Geometry check sheet. Reference: the model listing, model coordinates, mm. A direction names the side the tool comes from. Coordinates: 2 decimals unless noted, no trailing zeros. Loops run counter-clockwise (first coordinate to the right, second up) from the corner with the lowest first, then second, coordinate; pieces in that order, holes last.
from build123d import *

# Parameters (mm, degrees)
SM_BASE_FLANGE_1_DEPTH   = 41
SKETCH_9_R               = 2.5
CUT_EXTRUDE_4_DEPTH      = 61.6465168
CUT_EXTRUDE_5_DEPTH      = 78.103826105
CUT_EXTRUDE_5_DEPTH_BACK = 78.103826105
SKETCH_10_R              = 2.5


# Sheet-metal steps are written as plain solids
with BuildPart() as part:
    # Sketch 1 → Базовая кромка1 (new body)
    with BuildSketch(Plane.XY):
        with BuildLine():
            Line((-25, 30), (-25, 1))
            ThreePointArc((-25, 1), (-24.707106781, 0.292893219), (-24, 0))
            Line((-24, 0), (24, 0))
            ThreePointArc((24, 0), (24.707106781, 0.292893219), (25, 1))
            Line((25, 1), (25, 30))
            Line((25, 30), (29, 30))
            Line((29, 30), (29, 1))
            ThreePointArc((29, 1), (27.535533906, -2.535533906), (24, -4))
            Line((24, -4), (-24, -4))
            ThreePointArc((-24, -4), (-27.535533906, -2.535533906), (-29, 1))
            Line((-29, 1), (-29, 30))
            Line((-29, 30), (-25, 30))
        make_face()
    extrude(amount=SM_BASE_FLANGE_1_DEPTH)

    # Эскиз9 → Вырез-Вытянуть4 (cut, through all)
    with BuildSketch(Plane.XZ.offset(4)):
        with Locations((-18, 20.5)):
            Circle(SKETCH_9_R)
        with Locations((-9, 36.088457268)):
            Circle(SKETCH_9_R)
        with Locations((9, 36.088457268)):
            Circle(SKETCH_9_R)
        with Locations((18, 20.5)):
            Circle(SKETCH_9_R)
        with Locations((9, 4.911542732)):
            Circle(SKETCH_9_R)
        with Locations((-9, 4.911542732)):
            Circle(SKETCH_9_R)
    extrude(amount=-CUT_EXTRUDE_4_DEPTH, mode=Mode.SUBTRACT)

    # Эскиз10 → Вырез-Вытянуть5 (cut, two sides: drawn at the far end of the back side and taken through both)
    with BuildSketch(Plane(origin=(29, 0, 0), x_dir=(0, 0, -1), z_dir=(1, 0, 0)).offset(-CUT_EXTRUDE_5_DEPTH_BACK)):
        with Locations((-33, 25)):
            Circle(SKETCH_10_R)
        with Locations((-20.5, 25)):
            Circle(SKETCH_10_R)
        with Locations((-8, 25)):
            Circle(SKETCH_10_R)
        with Locations((-20.5, 12.5)):
            Circle(SKETCH_10_R)
    extrude(amount=CUT_EXTRUDE_5_DEPTH + CUT_EXTRUDE_5_DEPTH_BACK, mode=Mode.SUBTRACT)


solid = part.part
1) Mould release check, pull along X, two halves, no side actions. Record for faces 3 (the cylindrical face through (16, -2, 22)), 4 (the cylindrical face through (-27, -3, 20)), 5 (the flat face through (0, -1, 0)): +X half, -X half, draft (parallel to the pull), parting line (faces both ways), or undercut.
Data:
face 3: undercut
face 4: -X half
face 5: draft
2) Access from +Z, -Z, +X, -X, +Y, -Y to the whole of each face (thin tool, end or side, straight path). Record for faces 1 (the cylindrical face through (27, 11, 22.5)), 2 (the flat face through (25, 15.3, 20.2)).
Data:
face 1: +X, -X
face 2: +Z, -Z, +Y
3) Section check A-A on z = 9.5. Record the cut outline in (x, y).
Data:
outline: (-29, 1) arc R5 ccw to (-24, -4) - (24, -4) arc R5 ccw to (29, 1) - (29, 23) - (25, 23) - (25, 1) arc R1 cw to (24, 0) - (-24, 0) arc R1 cw to (-25, 1) - (-25, 23) - (-29, 23) - close; (-29, 27) - (-25, 27) - (-25, 30) - (-29, 30) - close; (25, 27) - (29, 27) - (29, 30) - (25, 30) - close
4) Section check B-B on x = 18. Record the cut outline in (y, z).
Data:
outline: (-4, 0) - (0, 0) - (0, 18) - (-4, 18) - close; (-4, 23) - (0, 23) - (0, 41) - (-4, 41) - close
5) Section check D-D on y = 13.5. Record the cut outline in (x, z).
Data:
outline: (-29, 0) - (-25, 0) - (-25, 18.21) - (-29, 18.21) - close; (-29, 22.79) - (-25, 22.79) - (-25, 41) - (-29, 41) - close; (25, 0) - (29, 0) - (29, 18.21) - (25, 18.21) - close; (25, 22.79) - (29, 22.79) - (29, 41) - (25, 41) - close
6) Section check C-C on y = 19. Record the cut outline in (x, z), and give its area (3 significant figures).
Data:
outline: (-29, 0) - (-25, 0) - (-25, 41) - (-29, 41) - close; (25, 0) - (29, 0) - (29, 41) - (25, 41) - close
area: 328 mm2
7) Depth check by flat-ended pin: pin 1 (3 mm diameter, centred on x = 9, z = 36.09, fed in from -Y); pin 2 (3 mm diameter, centred on x = 10, z = 34.5, fed in from +Y). Enter the tip coordinate at first touch or a pass-through.
Data:
pin 1: passes through
pin 2: stops at y = 0
8) Material ranges on probe 1 along Z at (x, y) = (-28.05, 25); probe 2 along Z at (x, y) = (9, -1); probe 3 along X at (y, z) = (19, 35.5), recorded low to high.
Data:
probe 1: z = 0 to 5.5, 10.5 to 18, 23 to 30.5, 35.5 to 41
probe 2: z = 0 to 2.41, 7.41 to 33.59, 38.59 to 41
probe 3: x = -29 to -25, 25 to 29
